Print and shaded views of the part. All mm, measured from the part's lowest x, y and z. A direction names the side the tool comes from. Coordinates: 2 decimals unless noted, no trailing zeros. Write each loop counter-clockwise with the first axis right and the second up, starting at its lowest first coordinate (ties: lowest second). Pieces come first, ordered by that corner, then holes. Notation, with made-up numbers: (4.5, 75) -> (37.5, 75) arc R20 cw to (37.5, 109) -> close; hole circle Ø11 at (11, 19.25). An arc over 180 degrees is marked (long way). Write item = value, one per line.
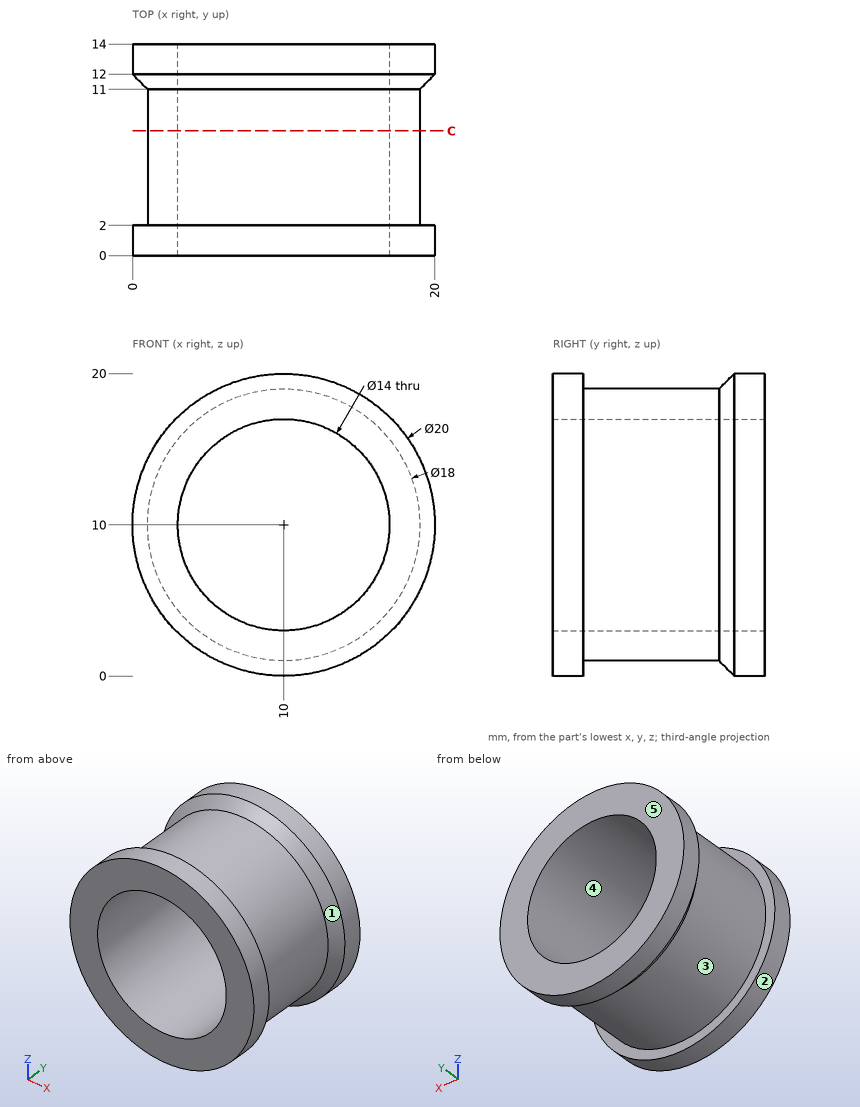
Q1. Mould opens along Z. For the marked faces 3, 4 and 5 say: released by +Z, released by -Z, zero draft, split by the parting line, or undercut.
Model answer:
face_3 = split by the parting line
face_4 = undercut
face_5 = zero draft
Q2. Probe line 1 (X direction, y = 3.75, z = 10); line 2 (X direction, y = 11.5, z = 10); line 3 (Z direction, x = 6.75, y = 7). List the from-to ranges inside material, lowest first. Write a range as from..to.
Model answer:
line_1 = 1..3, 17..19
line_2 = 0.5..3, 17..19.5
line_3 = 1.61..3.8, 16.2..18.39
Q3. Pin check, flat tips, straight feed: pin 1 (1.5 mm diameter, centred on x = 11, y = 3.5, fed in from -Z); pin 2 (4 mm diameter, centred on x = 7.5, y = 5.5, fed in from +Z); pin 3 (5 mm diameter, centred on x = 14.5, y = 8.5, fed in from +Z) (3 decimals). Stop position of each tip, or through.
Model answer:
pin_1 = 1
pin_2 = 18.99
pin_3 = 18.775
Q4. Saw through at C-C on y = 8.25. Give the cut face in (x, z).
Model answer:
outline = circle Ø18 at (10, 10); hole circle Ø14 at (10, 10)
Q5. Which spindle directions (+Z, -Z, +X, -X, +Y, -Y) get a long thin tool onto all of the face, cutting with end or side? Do the marked faces 1 and 2. Say none if no direction does.
Model answer:
face_1 = none
face_2 = +Y, -Y
